```python
from build123d import *

# Parameters (mm, degrees)
SKETCH1_R           = 2.250000000000002
SKETCH1_R_2         = 2.249999999999999
SKETCH1_R_3         = 2.6000000000000005
SKETCH1_R_4         = 2.600000000000003
BOSS_EXTRUDE1_DEPTH = 2.5
BOSS_EXTRUDE2_DEPTH = 7
CUT_EXTRUDE1_DEPTH  = 78.57966290553851
FILLET1_R           = 2


with BuildPart() as part:
    # Sketch1 → Boss-Extrude1 (new body)
    with BuildSketch(Plane.XY):
        with BuildLine():
            Line((-24.24262981574538, 11.568676716917917), (-7.792629815745428, 11.568676716917919))
            ThreePointArc((-7.792629815745428, 11.568676716917919), (-6.024862862779042, 12.30090976395155), (-5.292629815745411, 14.068676716917937))
            Line((-5.292629815745411, 14.068676716917937), (-5.2926298157454115, 24.208689532378564))
            ThreePointArc((-5.2926298157454115, 24.208689532378564), (-4.5603967687117795, 25.976456485344933), (-2.7926298157454106, 26.70868953237856))
            Line((-2.7926298157454106, 26.70868953237856), (-0.7926298157454105, 26.70868953237856))
            ThreePointArc((-0.7926298157454105, 26.70868953237856), (0.975137137220956, 25.97645648534493), (1.7073701842545899, 24.208689532378564))
            Line((1.7073701842545899, 24.208689532378564), (1.707370184254591, 14.068676716917937))
            ThreePointArc((1.707370184254591, 14.068676716917937), (2.439603231288222, 12.30090976395155), (4.207370184254609, 11.568676716917919))
            Line((4.207370184254609, 11.568676716917919), (15.807370184254571, 11.568676716917919))
            ThreePointArc((15.807370184254571, 11.568676716917919), (17.575137137220956, 12.300909763951552), (18.307370184254587, 14.068676716917935))
            Line((18.307370184254587, 14.068676716917935), (18.30737018425459, 24.208689532378564))
            ThreePointArc((18.30737018425459, 24.208689532378564), (19.039603231288222, 25.976456485344933), (20.80737018425459, 26.708689532378564))
            Line((20.80737018425459, 26.708689532378564), (22.80737018425459, 26.708689532378568))
            ThreePointArc((22.80737018425459, 26.708689532378568), (24.575137137220963, 25.976456485344936), (25.307370184254594, 24.208689532378564))
            Line((25.307370184254594, 24.208689532378564), (25.307370184254594, 14.068676716917937))
            ThreePointArc((25.307370184254594, 14.068676716917937), (26.039603231288226, 12.300909763951552), (27.80737018425461, 11.568676716917919))
            Line((27.80737018425461, 11.568676716917919), (44.25737018425458, 11.568676716917917))
            ThreePointArc((44.25737018425458, 11.568676716917917), (45.67158374662769, 10.982890279291011), (46.2573701842546, 9.568676716917901))
            Line((46.2573701842546, 9.568676716917901), (46.25737018425459, -1.4313232830820677))
            ThreePointArc((46.25737018425459, -1.4313232830820677), (45.67158374662768, -2.845536845455177), (44.257370184254576, -3.431323283082082))
            Line((44.257370184254576, -3.431323283082082), (-24.242629815745374, -3.431323283082082))
            ThreePointArc((-24.242629815745374, -3.431323283082082), (-25.656843378118484, -2.8455368454551784), (-26.242629815745392, -1.4313232830820677))
            Line((-26.242629815745392, -1.4313232830820677), (-26.2426298157454, 9.568676716917903))
            ThreePointArc((-26.2426298157454, 9.568676716917903), (-25.65684337811849, 10.982890279291013), (-24.24262981574538, 11.568676716917917))
        make_face()
        with Locations((38.7573701842546, 4.068676716917918)):
            Circle(SKETCH1_R, mode=Mode.SUBTRACT)
        with Locations((19.757370184254597, 4.068676716917918)):
            Circle(SKETCH1_R_2, mode=Mode.SUBTRACT)
        with Locations((0.7573701842545979, 4.068676716917918)):
            Circle(SKETCH1_R_2, mode=Mode.SUBTRACT)
        with Locations((-1.7926298157454108, 23.50868953237856)):
            Circle(SKETCH1_R_3, mode=Mode.SUBTRACT)
        with Locations((21.80737018425459, 23.508689532378565)):
            Circle(SKETCH1_R_4, mode=Mode.SUBTRACT)
        with BuildLine():
            Line((-22.24262981574538, 10.568676716917917), (-7.242629815745397, 10.56867671691792))
            ThreePointArc((-7.242629815745397, 10.56867671691792), (-5.8284162533723025, 9.982890279291016), (-5.2426298157453965, 8.56867671691792))
            Line((-5.2426298157453965, 8.56867671691792), (-5.242629815745396, -0.43132328308208134))
            ThreePointArc((-5.242629815745396, -0.43132328308208134), (-5.828416253372301, -1.8455368454551766), (-7.242629815745396, -2.4313232830820817))
            Line((-7.242629815745396, -2.4313232830820817), (-22.24262981574538, -2.431323283082082))
            ThreePointArc((-22.24262981574538, -2.431323283082082), (-23.65684337811849, -1.8455368454551762), (-24.242629815745396, -0.43132328308206774))
            Line((-24.242629815745396, -0.43132328308206774), (-24.242629815745396, 8.568676716917903))
            ThreePointArc((-24.242629815745396, 8.568676716917903), (-23.65684337811849, 9.982890279291013), (-22.24262981574538, 10.568676716917917))
        make_face(mode=Mode.SUBTRACT)
    extrude(amount=BOSS_EXTRUDE1_DEPTH)

    # Sketch2 → Boss-Extrude2 (add)
    with BuildSketch(Plane(origin=(0, 0, 0), x_dir=(-1, 0, 0), z_dir=(0, 0, -1))):
        with BuildLine():
            Line((-44.2573701842546, 11.591990827848472), (24.242629815745396, 11.591990827848472))
            ThreePointArc((24.242629815745396, 11.591990827848472), (25.65684337811849, 11.006204390221566), (26.2426298157454, 9.591990827848472))
            Line((26.2426298157454, 9.591990827848472), (26.2426298157454, -1.408009172151513))
            ThreePointArc((26.2426298157454, -1.408009172151513), (25.65684337811849, -2.8222227345246234), (24.24262981574538, -3.4080091721515275))
            Line((24.24262981574538, -3.4080091721515275), (-44.25737018425458, -3.4080091721515275))
            ThreePointArc((-44.25737018425458, -3.4080091721515275), (-45.67158374662769, -2.8222227345246225), (-46.2573701842546, -1.4080091721515136))
            Line((-46.2573701842546, -1.4080091721515136), (-46.2573701842546, 9.591990827848472))
            ThreePointArc((-46.2573701842546, 9.591990827848472), (-45.67158374662769, 11.006204390221567), (-44.2573701842546, 11.591990827848472))
        make_face()
        with BuildLine():
            Line((7.242629815745404, 10.591990827848473), (22.242629815745403, 10.591990827848472))
            ThreePointArc((22.242629815745403, 10.591990827848472), (23.6568433781185, 10.006204390221566), (24.242629815745403, 8.591990827848472))
            Line((24.242629815745403, 8.591990827848472), (24.242629815745403, -0.4080091721515276))
            ThreePointArc((24.242629815745403, -0.4080091721515276), (23.6568433781185, -1.8222227345246227), (22.242629815745403, -2.408009172151528))
            Line((22.242629815745403, -2.408009172151528), (7.2426298157454045, -2.4080091721515275))
            ThreePointArc((7.2426298157454045, -2.4080091721515275), (5.8284162533723105, -1.8222227345246227), (5.242629815745405, -0.40800917215152854))
            Line((5.242629815745405, -0.40800917215152854), (5.242629815745403, 8.591990827848472))
            ThreePointArc((5.242629815745403, 8.591990827848472), (5.828416253372307, 10.006204390221567), (7.242629815745404, 10.591990827848473))
        make_face(mode=Mode.SUBTRACT)
    extrude(amount=BOSS_EXTRUDE2_DEPTH)

    # Sketch3 → Cut-Extrude1 (cut, through all)
    with BuildSketch(Plane.ZY.offset(26.242629815745392)):
        Polygon((2.5, 11.568676716917924), (1.25, -3.4313232830820675), (2.5, -3.431323283082067), align=None)
    extrude(amount=-CUT_EXTRUDE1_DEPTH, mode=Mode.SUBTRACT)

    # Fillet1
    # the kernel refuses this fillet: 2 mm, written as the material it takes off along each edge
    with BuildSketch(Plane(origin=(-24.24262981574539, 9.591990827848464, -7), x_dir=(-3.55e-15, 1, 0), z_dir=(1, 3.55e-15, 0))) as fillet1_piece_1:
        with BuildLine():
            CenterArc((2.000000000000009 - FILLET1_R, FILLET1_R), FILLET1_R, 270, 90)
            Line((2.000000000000009 - FILLET1_R, 0), (2.000000000000009, 0))
            Line((2.000000000000009, 0), (2.000000000000009, FILLET1_R))
        make_face()
    revolve(axis=Axis((-24.24262981574539, 9.591990827848464, -7), (0, 0, 1)), revolution_arc=89.99999999999959, mode=Mode.SUBTRACT)
    with BuildSketch(Plane(origin=(-26.2426298157454, 9.591990827848472, -7), x_dir=(0, 0, 1), z_dir=(0, -1, 0))) as fillet1_piece_2:
        with BuildLine():
            CenterArc((FILLET1_R, -FILLET1_R), FILLET1_R, 90, 89.99999999999989)
            Line((0, -FILLET1_R), (0, 0))
            Line((0, 0), (FILLET1_R, 0))
        make_face()
    extrude(amount=10.999999999999984, mode=Mode.SUBTRACT)
    with BuildSketch(Plane(origin=(-24.242629815745396, -1.4080091721515238, -7), x_dir=(-1, 5.33e-15, 0), z_dir=(5.33e-15, 1, 0))) as fillet1_piece_3:
        with BuildLine():
            CenterArc((2.0000000000000036 - FILLET1_R, FILLET1_R), FILLET1_R, 270.0000000000001, 89.99999999999989)
            Line((2.0000000000000036 - FILLET1_R, 0), (2.0000000000000036, 0))
            Line((2.0000000000000036, 0), (2.0000000000000036, FILLET1_R))
        make_face()
    revolve(axis=Axis((-24.242629815745396, -1.4080091721515238, -7), (0, 0, 1)), revolution_arc=90.00000000000071, mode=Mode.SUBTRACT)
    with BuildSketch(Plane(origin=(-24.24262981574538, -3.4080091721515275, -7), x_dir=(0, 1, 0), z_dir=(1, 0, 0))) as fillet1_piece_4:
        with BuildLine():
            CenterArc((FILLET1_R, FILLET1_R), FILLET1_R, 180, 90)
            Line((0, FILLET1_R), (0, 0))
            Line((0, 0), (FILLET1_R, 0))
        make_face()
    extrude(amount=68.49999999999997, mode=Mode.SUBTRACT)
    with BuildSketch(Plane(origin=(44.25737018425459, -1.408009172151522, -7), x_dir=(-3.55e-15, -1, 0), z_dir=(-1, 3.55e-15, 0))) as fillet1_piece_5:
        with BuildLine():
            CenterArc((2.000000000000006 - FILLET1_R, FILLET1_R), FILLET1_R, 270, 90)
            Line((2.000000000000006, FILLET1_R), (2.000000000000006, 0))
            Line((2.000000000000006, 0), (2.000000000000006 - FILLET1_R, 0))
        make_face()
    revolve(axis=Axis((44.25737018425459, -1.408009172151522, -7), (0, 0, 1)), revolution_arc=90.00000000000044, mode=Mode.SUBTRACT)
    with BuildSketch(Plane(origin=(46.2573701842546, -1.4080091721515136, -7), x_dir=(-3.55e-15, 0, 1), z_dir=(0, 1, 0))) as fillet1_piece_6:
        with BuildLine():
            CenterArc((FILLET1_R, -FILLET1_R), FILLET1_R, 90.0000000000002, 89.9999999999998)
            Line((7.11e-15, -FILLET1_R), (0, 0))
            Line((0, 0), (FILLET1_R, 0))
        make_face()
    extrude(amount=10.999999999999986, mode=Mode.SUBTRACT)
    with BuildSketch(Plane(origin=(44.2573701842546, 9.591990827848468, -7), x_dir=(1, 1.78e-15, 0), z_dir=(1.78e-15, -1, 0))) as fillet1_piece_7:
        with BuildLine():
            CenterArc((2 - FILLET1_R, FILLET1_R), FILLET1_R, 270, 90)
            Line((2, FILLET1_R), (2, 0))
            Line((2, 0), (2 - FILLET1_R, 0))
        make_face()
    revolve(axis=Axis((44.2573701842546, 9.591990827848468, -7), (0, 0, 1)), revolution_arc=89.9999999999999, mode=Mode.SUBTRACT)
    with BuildSketch(Plane(origin=(44.2573701842546, 11.591990827848472, -7), x_dir=(0, 0, 1), z_dir=(-1, 0, 0))) as fillet1_piece_8:
        with BuildLine():
            CenterArc((FILLET1_R, -FILLET1_R), FILLET1_R, 90, 90)
            Line((0, -FILLET1_R), (0, 0))
            Line((0, 0), (FILLET1_R, 0))
        make_face()
    extrude(amount=68.5, mode=Mode.SUBTRACT)


solid = part.part
```
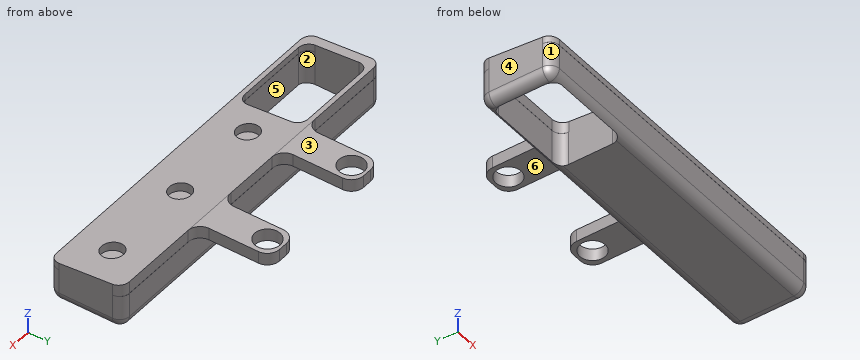
Model file for the job. Use its own axes, mm. Face numbers are marked on the shaded views. A direction names the side the tool comes from. Give positions to 0.01 mm unless a question says otherwise; leave off trailing zeros. Loops run counter-clockwise (first coordinate to the right, second up) from the corner with the lowest first, then second, coordinate; pieces in that order, holes last. Notation, with made-up numbers: (29.25, 41.25) -> (56.25, 41.25) arc R21 cw to (56.25, 47.25) -> close; hole circle Ø10 at (63.5, 42). An arc over 180 degrees is marked (long way). Use CSV: the item, a comma, the result in double quotes. Start each with the question number.
1) Tool access for the marked faces 4, 5 and 6: list every direction of +Z, -Z, +X, -X, +Y, -Y with a clear straight run to the whole face (end or side of a thin tool).
2) Flat gauge pins, fed straight in: pin 1 Ø2 at (x, y) = (28, 19) entering from -Z; pin 2 Ø5.5 at (x, z) = (-16.5, -4) entering from -Y; pin 3 Ø2 at (x, y) = (1.5, 3.5) entering from +Z; pin 4 Ø3.5 at (x, y) = (38, 3) entering from +Z. Where does each tip first touch, or does it go through?
3) Mould opens along X. For the marked faces 1, 2 and 3 say: released by +X, released by -X, zero draft, split by the parting line, or undercut.
4) Slice it at B-B on y = 19.5. Give the cut face in (x, z), plus the area to 3 significant figures.
5) Wall check: line 1 (X direction, y = 0, z = -4.5); line 2 (Y direction, x = -18, z = -1.5); line 3 (Y direction, x = 24.5, z = -2). Give the ranges that are in metal, low to high.
6) Slice it at C-C on z = -1.75. Give the cut face in (x, y), plus the area to 4 significant figures.
Computed values:
1,face 4,"+Z, -Z, -X, +Y, -Y"
1,face 5,"+Z, -Z"
1,face 6,"-Z, +X, -X, +Y"
2,pin 1,"passes through"
2,pin 2,"stops at y = -3.41"
2,pin 3,"stops at z = 0"
2,pin 4,"stops at z = 1.86"
3,face 1,"released by -X"
3,face 2,"undercut"
3,face 3,"zero draft"
4,outline,"(-5.29, 0) -> (1.71, 0) -> (1.71, 2.5) -> (-5.29, 2.5) -> close; (18.31, 0) -> (25.31, 0) -> (25.31, 2.5) -> (18.31, 2.5) -> close"
4,area,"35.0 mm^2"
5,line 1,"x = -26.24 to -24.24, -5.24 to 46.26"
5,line 2,"y = -3.41 to -2.41, 10.59 to 11.59"
5,line 3,"y = -3.41 to 11.59"
6,outline,"(-26.24, -1.41) arc R2 ccw to (-24.24, -3.41) -> (44.26, -3.41) arc R2 ccw to (46.26, -1.41) -> (46.26, 9.59) arc R2 ccw to (44.26, 11.59) -> (-24.24, 11.59) arc R2 ccw to (-26.24, 9.59) -> close; hole (-24.24, -0.41) arc R2 ccw to (-22.24, -2.41) -> (-7.24, -2.41) arc R2 ccw to (-5.24, -0.41) -> (-5.24, 8.59) arc R2 ccw to (-7.24, 10.59) -> (-22.24, 10.59) arc R2 ccw to (-24.24, 8.59) -> close"
6,area,"840.5 mm^2"
